Geometry: final body of the model. Coordinates: model frame, mm. A direction names the side the tool comes from. Give positions to 0.01 mm unless a question says otherwise; leave off trailing zeros. Loops run counter-clockwise (first coordinate to the right, second up) from the corner with the lowest first, then second, coordinate; pieces in that order, holes last. Notation, with made-up numbers: (-6, 69.25) - (28, 69.25) arc R14 cw to (28, 82.25) - close; hole circle Ø1 at (61.5, -39). An arc over 180 degrees is marked (long way). Use one line per item in the form item = value.
```python
from build123d import *

# Parameters (mm, degrees)
SKETCH1_W           = 222.25
SKETCH1_H           = 222.25
BOSS_EXTRUDE1_DEPTH = 5.15
SKETCH2_W           = 26.49375
SKETCH2_H           = 10.3
SKETCH2_W_2         = 10.3
SKETCH2_H_2         = 27.78125
CUT_EXTRUDE1_DEPTH  = 315.351153171
BOSS_EXTRUDE2_DEPTH = 5.15
CUT_EXTRUDE2_DEPTH  = 329.096441614


with BuildPart() as part:
    # Sketch1 → Boss-Extrude1 (new body)
    with BuildSketch(Plane(origin=(0, 0, 0), x_dir=(1, 0, 0), z_dir=(0, 1, 0))):
        with Locations((111.125, 111.125)):
            Rectangle(SKETCH1_W, SKETCH1_H)
    extrude(amount=BOSS_EXTRUDE1_DEPTH)

    # Sketch2 → Cut-Extrude1 (cut, through all)
    with BuildSketch(Plane(origin=(0, 5.15, 0), x_dir=(1, 0, 0), z_dir=(0, 1, 0))):
        with Locations((182.509375, 5.15)):
            Rectangle(SKETCH2_W, SKETCH2_H)
        with Locations((129.521875, 5.15)):
            Rectangle(SKETCH2_W, SKETCH2_H)
        with Locations((76.534375, 5.15)):
            Rectangle(SKETCH2_W, SKETCH2_H)
        with Locations((23.546875, 5.15)):
            Rectangle(SKETCH2_W, SKETCH2_H)
        Polygon((0, 0), (10.3, 0), (10.3, 10.3), (10.3, 27.78125), (0, 27.78125), align=None)
        with Locations((5.15, 69.453125)):
            Rectangle(SKETCH2_W_2, SKETCH2_H_2)
        with Locations((5.15, 125.015625)):
            Rectangle(SKETCH2_W_2, SKETCH2_H_2)
        with Locations((5.15, 180.578125)):
            Rectangle(SKETCH2_W_2, SKETCH2_H_2)
    extrude(amount=-CUT_EXTRUDE1_DEPTH, mode=Mode.SUBTRACT)

    # Sketch3 → Boss-Extrude2 (add)
    with BuildSketch(Plane(origin=(0, 5.15, 0), x_dir=(1, 0, 0), z_dir=(0, 1, 0))):
        Polygon((73.025, 222.25), (60.325, 241.3), (161.925, 241.3), (149.225, 222.25), align=None)
    extrude(amount=-BOSS_EXTRUDE2_DEPTH)

    # Sketch4 → Cut-Extrude2 (cut, through all)
    with BuildSketch(Plane(origin=(0, 5.15, 0), x_dir=(1, 0, 0), z_dir=(0, 1, 0))):
        Polygon((222.25, 73.025), (203.2, 60.325), (203.2, 161.925), (222.25, 149.225), align=None)
    extrude(amount=-CUT_EXTRUDE2_DEPTH, mode=Mode.SUBTRACT)


solid = part.part
```
(1) Access query for faces 4 (the face through (5, 3, -166.688)), 5 (the face through (185, 3, -222.25)), 6 (the face through (212.858, 2.611, -66.764)). Directions: +Z, -Z, +X, -X, +Y, -Y. A direction counts if a zero-diameter tool reaches every point of the face in a straight line with its end or side. Return the directions, or none.
Solution:
face_4 = -X, +Y, -Y
face_5 = +X, +Y, -Y
face_6 = +Y, -Y
(2) Cut plane C-C (x = 56.5). Return the cut outline in (y, z), plus the area to 3 significant figures.
Solution:
outline = (0, -222.25) - (5.15, -222.25) - (5.15, 0) - (0, 0) - close
area = 1,140 mm2
(3) Pin query (flat end, axial travel): P1, Ø1.5, axis at x = 173.5, y = 1.5, coming from the -Z side; P2, Ø2, axis at x = 165.5, y = 3, coming from the +Z side; P3, Ø2.5, axis at y = 1.5, z = -175, coming from the -X side; P4, Ø1.5, axis at x = 21.5, y = 2, coming from the +Z side. Return the tip coordinate at first contact, or that it passes through.
Solution:
P1 = -222.25
P2 = 0
P3 = 10.3
P4 = -10.3
(4) Cut plane D-D (z = -133). Return the cut outline in (x, y), plus the area to 3 significant figures.
Solution:
outline = (10.3, 0) - (203.2, 0) - (203.2, 5.15) - (10.3, 5.15) - close
area = 993 mm2
(5) Material intervals for L1, parallel to Z at x = 178, y = 0.8; L2, parallel to Z at x = 86, y = 0.8; L3, parallel to X at y = 3.35, z = -119, sorted ascending. Write a range as from..to.
Solution:
L1 = -222.25..-10.3
L2 = -241.3..-10.3
L3 = 10.3..203.2
(6) Cut plane B-B (x = 152). Return the cut outline in (y, z).
Solution:
outline = (0, -241.3) - (5.15, -241.3) - (5.15, -226.41) - (0, -226.41) - close; (0, -222.25) - (5.15, -222.25) - (5.15, 0) - (0, 0) - close
(7) Cut plane A-A (z = -159). Return the cut outline in (x, y).
Solution:
outline = (0, 0) - (203.2, 0) - (203.2, 5.15) - (0, 5.15) - close; (207.59, 0) - (222.25, 0) - (222.25, 5.15) - (207.59, 5.15) - close
(8) Pull-direction query (Z, two-part tool) for faces 1 (the face through (10.3, 3, -19)), 2 (the face through (5, 3, -138.906)), 3 (the face through (182, 3, -10.3)); classes: released by +Z, released by -Z, zero draft, split by the parting line, or undercut.
Solution:
face_1 = zero draft
face_2 = undercut
face_3 = released by +Z
